```python
from build123d import *

# Parameters (mm, degrees)
EXTRUDE_1_DEPTH     = 76
FILLET_1_R          = 38
RIB_1_REACH         = 148.127
SKETCH_4_WALL_W     = 393.877609006
SKETCH_4_WALL_H     = 5
RIB_START           = -5
RIB_2_DEPTH         = 5
SKETCH_7_R          = 2.5
CUT_EXTRUDE_1_DEPTH = 10
FILLET_2_R          = 2
CHAMFER_1_SIZE      = 10
CHAMFER_1_SIZE2     = 5
FILLET_3_R          = 2
FILLET_4_R          = 2
SKETCH_8_R          = 20
CUT_EXTRUDE_2_DEPTH = 5
EXTRUDE_START       = 25
SKETCH_8_6_R        = 25
SKETCH_8_6_R_2      = 20
EXTRUDE_4_DEPTH     = 25
FILLET_5_R          = 5
SKETCH_13_R         = 4
CUT_EXTRUDE_3_DEPTH = 76
SKETCH_14_R         = 4
CUT_EXTRUDE_4_DEPTH = 76


with BuildPart() as part:
    # Эскиз3 → Бобышка-Вытянуть1 (new body)
    with BuildSketch(Plane.XY):
        Polygon((76, 0), (0, 0), (0, 5), (71, 5), (71, 99), (76, 99), align=None)
    extrude(amount=EXTRUDE_1_DEPTH)

    # Скругление1
    fillet_1_edges = [part.edges().sort_by_distance(p)[0] for p in [
        (0, 2.5, 0),
        (0, 2.5, 76),
    ]]
    fillet(fillet_1_edges, radius=FILLET_1_R - 0.0001)  # a hair under: the kernel refuses the full size

    # Эскиз4 wall → Ребро1 (add, up to next)
    with BuildSketch(Plane(origin=(54.5, 52, 76), x_dir=(-0.331244504731, -0.94354495287, 0), z_dir=(0.94354495287, -0.331244504731, 0)), mode=Mode.PRIVATE) as rib_1_sk1:
        with Locations((0, 2.5)):
            Rectangle(SKETCH_4_WALL_W, SKETCH_4_WALL_H)
    rib_1_tool1 = extrude(rib_1_sk1.sketch, amount=RIB_1_REACH, mode=Mode.PRIVATE) - part.part
    add(rib_1_tool1.solids().sort_by_distance((54.5, 52, 76))[0])

    # Ребро2: read off the stored shape, not the designer's step
    # Ребро2 outline → Ребро2 (add)
    with BuildSketch(Plane(origin=(0, 0, 0), x_dir=(-1, 0, 0), z_dir=(0, 0, -1)).offset(RIB_START)):
        Polygon((-38, 5), (-71, 99), (-71, 5), align=None)
    extrude(amount=RIB_2_DEPTH)

    # Эскиз7 → Вырез-Вытянуть1 (cut)
    with BuildSketch(Plane(origin=(0, 5, 0), x_dir=(1, 0, 0), z_dir=(0, 1, 0))):
        with Locations(Location((20, -38, 0), (0, 0, 180))):
            Circle(SKETCH_7_R)
        with Locations(Location((29, -22.411542732, 0), (0, 0, 180))):
            Circle(SKETCH_7_R)
        with Locations(Location((47, -22.411542732, 0), (0, 0, 180))):
            Circle(SKETCH_7_R)
        with Locations(Location((56, -38, 0), (0, 0, 180))):
            Circle(SKETCH_7_R)
        with Locations(Location((47, -53.588457268, 0), (0, 0, 180))):
            Circle(SKETCH_7_R)
        with Locations(Location((29, -53.588457268, 0), (0, 0, 180))):
            Circle(SKETCH_7_R)
    extrude(amount=-CUT_EXTRUDE_1_DEPTH, mode=Mode.SUBTRACT)

    # Скругление2
    fillet_2_edges = [part.edges().sort_by_distance(p)[0] for p in [
        (76, 0, 38),
    ]]
    fillet(fillet_2_edges, radius=FILLET_2_R)

    # Фаска1
    chamfer_1_edges = [part.edges().sort_by_distance(p)[0] for p in [
        (71, 5, 38),
    ]]
    chamfer_1_side = [part.faces().sort_by_distance(p)[0] for p in [
        (71, 52, 38),
    ]]
    chamfer(chamfer_1_edges, length=CHAMFER_1_SIZE, length2=CHAMFER_1_SIZE2, reference=chamfer_1_side[0])

    # Скругление3
    fillet_3_edges = [part.edges().sort_by_distance(p)[0] for p in [
        (38, 5, 73.5),
        (38, 5, 2.5),
    ]]
    fillet(fillet_3_edges, radius=FILLET_3_R)

    # Скругление4
    fillet_4_edges = [part.edges().sort_by_distance(p)[0] for p in [
        (73.5, 99, 76),
        (73.5, 99, 0),
    ]]
    fillet(fillet_4_edges, radius=FILLET_4_R)

    # Эскиз8 → Вырез-Вытянуть2 (cut)
    with BuildSketch(Plane(origin=(76, 0, 0), x_dir=(0, 0, -1), z_dir=(1, 0, 0))):
        with Locations((-38, 50)):
            Circle(SKETCH_8_R)
    extrude(amount=-CUT_EXTRUDE_2_DEPTH, mode=Mode.SUBTRACT)

    # Эскиз8<6> → Бобышка-Вытянуть4 (add)
    with BuildSketch(Plane(origin=(76, 0, 0), x_dir=(0, 0, -1), z_dir=(1, 0, 0)).offset(EXTRUDE_START)):
        with Locations(Location((-38, 50, 0), (0, 0, 180))):
            Circle(SKETCH_8_6_R)
        with Locations((-38, 50)):
            Circle(SKETCH_8_6_R_2, mode=Mode.SUBTRACT)
    extrude(amount=-EXTRUDE_4_DEPTH)

    # Скругление5
    fillet_5_edges = [part.edges().sort_by_distance(p)[0] for p in [
        (76, 50, 13),
    ]]
    fillet(fillet_5_edges, radius=FILLET_5_R)

    # Эскиз13 → Вырез-Вытянуть3 (cut)
    with BuildSketch(Plane(origin=(0, 0, 0), x_dir=(-1, 0, 0), z_dir=(0, 0, -1))):
        with Locations((-91, 50)):
            Circle(SKETCH_13_R)
    extrude(amount=-CUT_EXTRUDE_3_DEPTH, mode=Mode.SUBTRACT)

    # Эскиз14 → Вырез-Вытянуть4 (cut)
    with BuildSketch(Plane(origin=(0, 99, 0), x_dir=(1, 0, 0), z_dir=(0, 1, 0))):
        with Locations(Location((91, -38, 0), (0, 0, 270))):
            Circle(SKETCH_14_R)
    extrude(amount=-CUT_EXTRUDE_4_DEPTH, mode=Mode.SUBTRACT)


solid = part.part
```
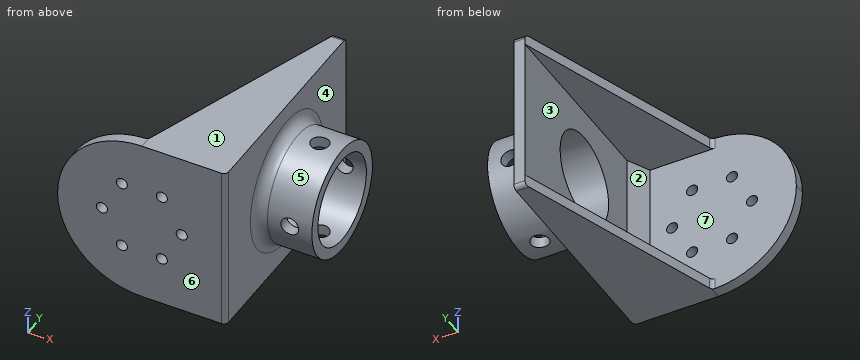
Here's how the part is built. I have some questions about the finished solid (model axes, mm). Face numbers are marked on the shaded views. A direction names the side the tool comes from. Round coordinates to 2 decimals unless told otherwise and drop trailing zeros. Write each loop counter-clockwise with the first axis right and the second up, starting at its lowest first coordinate (ties: lowest second). Pieces come first, ordered by that corner, then holes.
Q1. If we section it at B-B on x = 91: Write out the boundary of the cut face in (y, z).
Q2. If we section it at D-D on x = 47: Write out the boundary of the cut face in (y, z), plus the area to 3 significant figures.
Q3. Please list where these lines run through material, in increasing order: probe 1 along Z at (x, y) = (63.5, 19); probe 2 along X at (y, z) = (50, 16); probe 3 along Y at (x, z) = (56.5, 51).
Q4. Which directions (+Z, -Z, +X, -X, +Y, -Y) give clear straight access to the entire face, cutting with the end or side of a thin tool? Please do the marked faces 5, 6 and 7.
Q5. If we section it at C-C on y = 50: Write out the boundary of the cut face in (x, z).
Q6. If we mould it in two halves opening along Z, with no side actions, what happens to the marked faces 1, 2, 3 and 4? For each: +Z half, -Z half, draft (parallel to the pull), parting line (faces both ways), or undercut.
Q7. Will these pins go through, and if not, where does the flat tip stop? P1, Ø3, axis at x = 29, z = 53.59, coming from the -Y side; P2, Ø8, axis at x = 20, z = 38, coming from the +Y side; P3, Ø10.5, axis at x = 91, z = 38, coming from the -Y side; P4, Ø1.5, axis at y = 13.5, z = 11.5, coming from the -X side (3 decimals).
Q8. If we section it at A-A on x = 20: Write out the boundary of the cut face in (y, z), plus the area to 3 significant figures.
Answer below:
1. outline: (25.32, 34) arc R25 ccw to (46, 13.32) - (46, 18.4) arc R20 cw to (30.4, 34) - close; (25.32, 42) - (30.4, 42) arc R20 cw to (46, 57.6) - (46, 62.68) arc R25 ccw to start; (54, 13.32) arc R25 ccw to (74.68, 34) - (69.6, 34) arc R20 cw to (54, 18.4) - close; (54, 57.6) arc R20 cw to (69.6, 42) - (74.68, 42) arc R25 ccw to (54, 62.68) - close
2. outline: (0, 0) - (30.64, 0) - (30.64, 5) - (5, 5) - (5, 19.91) - (0, 19.91) - close; (0, 24.91) - (5, 24.91) - (5, 51.09) - (0, 51.09) - close; (0, 56.09) - (5, 56.09) - (5, 71) - (30.64, 71) - (30.64, 76) - (0, 76) - close
2. area: 586 mm2
3. probe 1: z = 0 to 5, 71 to 76
3. probe 2: x = 71 to 87, 95 to 101
3. probe 3: y = 0 to 5
4. face 5: +X
4. face 6: +Z, -Z, +X, -X, -Y
4. face 7: -X, +Y
5. outline: (53.8, 0) - (76, 0) - (76, 8) arc R5 cw to (81, 13) - (87, 13) - (87, 18) - (71, 18) - (71, 5) - (53.8, 5) - close; (53.8, 71) - (71, 71) - (71, 58) - (87, 58) - (87, 63) - (81, 63) arc R5 cw to (76, 68) - (76, 76) - (53.8, 76) - close; (95, 13) - (101, 13) - (101, 18) - (95, 18) - close; (95, 58) - (101, 58) - (101, 63) - (95, 63) - close
6. face 1: +Z half
6. face 2: undercut
6. face 3: undercut
6. face 4: draft
7. P1: passes through
7. P2: stops at y = 5
7. P3: stops at y = 25
7. P4: stops at x = 69.875
8. outline: (0, 4.53) - (5, 4.53) - (5, 35.5) - (0, 35.5) - close; (0, 40.5) - (5, 40.5) - (5, 71.47) - (0, 71.47) - close
8. area: 310 mm2
